The listing builds one solid part. Answer for the finished solid, in the listing's coordinates (mm). Face numbers are marked on the shaded views. A direction names the side the tool comes from. Give positions to 0.01 mm unless a question says otherwise; leave off trailing zeros. Write each loop counter-clockwise with the first axis right and the second up, starting at its lowest first coordinate (ties: lowest second). Pieces come first, ordered by that corner, then holes. Notation, with made-up numbers: (76, 53) - (129, 53) arc R33 cw to (129, 84) - close; hole circle Ø3 at (-34, 13.25). An arc over 180 degrees is marked (long way). Use a Markdown table: item, result. Add a question column.
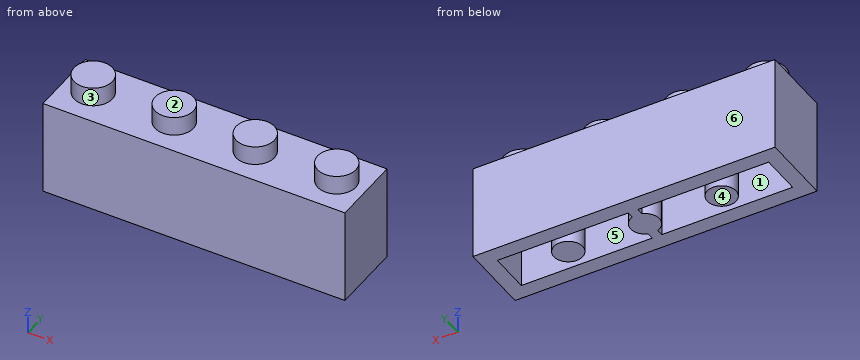
from build123d import *

# Parameters (mm, degrees)
F0_W     = 31.5
F0_H     = 7.45
F0_R     = 2
F1_DEPTH = 10
F2_DEPTH = 12
F3_R     = 1.5
F4_DEPTH = 9


with BuildPart() as f1:
    # F0 (on Top) → F1 (new body)
    with BuildSketch(Plane.XY):
        Rectangle(F0_W, F0_H)
        with Locations((-12.7, 0)):
            Circle(F0_R, mode=Mode.SUBTRACT)
        with Locations((-4.25, 0)):
            Circle(F0_R, mode=Mode.SUBTRACT)
        with Locations((4.2, 0)):
            Circle(F0_R, mode=Mode.SUBTRACT)
        with Locations((12.7, 0)):
            Circle(F0_R, mode=Mode.SUBTRACT)
    extrude(amount=F1_DEPTH)

    # F0 (on Top) → F2 (join)
    with BuildSketch(Plane.XY):
        with Locations((-12.7, 0)):
            Circle(F0_R)
        with Locations((-4.25, 0)):
            Circle(F0_R)
        with Locations((4.2, 0)):
            Circle(F0_R)
        with Locations((12.7, 0)):
            Circle(F0_R)
    extrude(amount=F2_DEPTH)

    # F3 (on face) → F4 (cut)
    with BuildSketch(Plane(origin=(0, 0, 0), x_dir=(1, 0, 0), z_dir=(0, 0, -1))):
        with BuildLine():
            Line((14.15, -2.125), (14.15, 2.125))
            Line((14.15, 2.125), (0.5, 2.125))
            Line((0.5, 2.125), (0.5, 1.414214))
            ThreePointArc((0.5, 1.414214), (1.224745, 0.866025), (1.5, 0))
            ThreePointArc((1.5, 0), (1.224745, -0.866025), (0.5, -1.414214))
            Line((0.5, -1.414214), (0.5, -2.125))
            Line((0.5, -2.125), (14.15, -2.125))
        make_face()
        with Locations((8, 0)):
            Circle(F3_R, mode=Mode.SUBTRACT)
        with BuildLine():
            Line((-0.5, 1.414214), (-0.5, 2.125))
            Line((-0.5, 2.125), (-14.15, 2.125))
            Line((-14.15, 2.125), (-14.15, -2.125))
            Line((-14.15, -2.125), (-0.5, -2.125))
            Line((-0.5, -2.125), (-0.5, -1.414214))
            ThreePointArc((-0.5, -1.414214), (-1.5, 0), (-0.5, 1.414214))
        make_face()
        with Locations((-8, 0)):
            Circle(F3_R, mode=Mode.SUBTRACT)
    extrude(amount=-F4_DEPTH, mode=Mode.SUBTRACT)


solid = f1.part
1. The part is cut by section B-B (x = -8). Give the vertices of the cut face in (y, z) (3 decimals), and give its area (4 significant figures).
2. The part is cut by section D-D (x = -11.5). Give the vertices of the cut face in (y, z) (3 decimals), and give its area (4 significant figures).
3. Consider L1, parallel to X at y = -2, z = 6.75; L2, parallel to X at y = 0, z = 6.5; L3, parallel to Y at x = -4, z = 4 (3 decimals). Determine where each line is inside the solid, lowest interval first. Write a range as [from, to].
4. The part is cut by section A-A (z = 4). Give the vertices of the cut face in (x, y) (3 decimals).
5. The part is cut by section C-C (y = 3.25). Give the vertices of the cut face in (x, z), and give its area (3 significant figures).
6. Which of the six approach directions +Z, -Z, +X, -X, +Y, -Y give full straight-line access (tool end or side, diameter ignored) to the marked faces 1, 2 and 3?
7. For a pull along Y with two mould halves and no side action, classify the marked faces 4, 5 and 6 as released by +Y, released by -Y, zero draft, split by the parting line, or undercut.
Check values:
| question | item | result |
|---|---|---|
| 1 | outline | (-3.725, 0) - (-2.125, 0) - (-2.125, 9) - (-1.5, 9) - (-1.5, 0) - (1.5, 0) - (1.5, 9) - (2.125, 9) - (2.125, 0) - (3.725, 0) - (3.725, 10) - (-3.725, 10) - close |
| 1 | area | 63.25 mm2 |
| 2 | outline | (-3.725, 0) - (-2.125, 0) - (-2.125, 9) - (2.125, 9) - (2.125, 0) - (3.725, 0) - (3.725, 10) - (1.6, 10) - (1.6, 12) - (-1.6, 12) - (-1.6, 10) - (-3.725, 10) - close |
| 2 | area | 42.65 mm2 |
| 3 | L1 | x = [-15.75, -14.15], [-0.5, 0.5], [14.15, 15.75] |
| 3 | L2 | x = [-15.75, -14.15], [-9.5, -6.5], [-1.5, 1.5], [6.5, 9.5], [14.15, 15.75] |
| 3 | L3 | y = [-3.725, -2.125], [2.125, 3.725] |
| 4 | outline | (-15.75, -3.725) - (15.75, -3.725) - (15.75, 3.725) - (-15.75, 3.725) - close; circle Ø3 at (-8, 0); circle Ø3 at (8, 0); hole (-14.15, -2.125) - (-0.5, -2.125) - (-0.5, -1.414) arc R1.5 cw to (-0.5, 1.414) - (-0.5, 2.125) - (-14.15, 2.125) - close; hole (0.5, -2.125) - (14.15, -2.125) - (14.15, 2.125) - (0.5, 2.125) - (0.5, 1.414) arc R1.5 cw to (1.5, 0) arc R1.5 cw to (0.5, -1.414) - close |
| 5 | outline | (-15.75, 0) - (15.75, 0) - (15.75, 10) - (-15.75, 10) - close |
| 5 | area | 315 mm2 |
| 6 | face 1 | -Z |
| 6 | face 2 | +Z, +X, -X, +Y, -Y |
| 6 | face 3 | +Z |
| 7 | face 4 | zero draft |
| 7 | face 5 | undercut |
| 7 | face 6 | released by +Y |
